```python
from build123d import *

# Parameters (mm, degrees)
SKETCH1_R               = 2
BOSS_EXTRUDE1_DEPTH     = 6
SKETCH1_3_W             = 26
SKETCH1_3_H             = 13
BOSS_EXTRUDE2_DEPTH     = 32
FILLET1_R               = 2.5
SKETCH2_R               = 9
CUT_EXTRUDE1_DEPTH      = 42.221960167
CUT_EXTRUDE2_REACH      = 48.971
CUT_EXTRUDE2_END_RADIUS = 9
SKETCH3_R               = 2
FILLET2_R               = 1


with BuildPart() as part:
    # Sketch1 → Boss-Extrude1 (new body)
    with BuildSketch(Plane(origin=(0, 0, 0), x_dir=(1, 0, 0), z_dir=(0, 1, 0))):
        with BuildLine():
            Line((-13, 0), (-22.5, 0))
            Line((-22.5, 0), (-22.5, -21))
            ThreePointArc((-22.5, -21), (-21.035533906, -24.535533906), (-17.5, -26))
            Line((-17.5, -26), (17.5, -26))
            ThreePointArc((17.5, -26), (21.035533906, -24.535533906), (22.5, -21))
            Line((22.5, -21), (22.5, 0))
            Line((22.5, 0), (13, 0))
            Line((13, 0), (13, -13))
            Line((13, -13), (-13, -13))
            Line((-13, -13), (-13, 0))
        make_face()
        with Locations(Location((0, -19.5, 0), (0, 0, 270))):
            Circle(SKETCH1_R, mode=Mode.SUBTRACT)
        with Locations(Location((-18, -6.5, 0), (0, 0, 270))):
            Circle(SKETCH1_R, mode=Mode.SUBTRACT)
        with Locations(Location((18, -6.5, 0), (0, 0, 270))):
            Circle(SKETCH1_R, mode=Mode.SUBTRACT)
    extrude(amount=BOSS_EXTRUDE1_DEPTH)

    # Sketch1<3> → Boss-Extrude2 (add)
    with BuildSketch(Plane(origin=(0, 0, 0), x_dir=(1, 0, 0), z_dir=(0, 1, 0))):
        with Locations((0, -6.5)):
            Rectangle(SKETCH1_3_W, SKETCH1_3_H)
    extrude(amount=BOSS_EXTRUDE2_DEPTH)

    # Fillet1
    fillet1_edges = [part.edges().sort_by_distance(p)[0] for p in [
        (-13, 32, 6.5),
        (13, 32, 6.5),
    ]]
    fillet(fillet1_edges, radius=FILLET1_R)

    # Sketch2 → Cut-Extrude1 (cut, through all)
    with BuildSketch(Plane.XY.offset(13)):
        with Locations((0, 19)):
            Circle(SKETCH2_R)
    extrude(amount=-CUT_EXTRUDE1_DEPTH, mode=Mode.SUBTRACT)

    # Cut-Extrude2: up to this cylinder (the profile starts outside it)
    cut_extrude2_end = Plane(origin=(0, 19, 6.5), z_dir=(0, 0, 1)) * Cylinder(CUT_EXTRUDE2_END_RADIUS, 116.942, mode=Mode.PRIVATE)
    # Sketch3 → Cut-Extrude2 (cut, up to the surface)
    with BuildSketch(Plane(origin=(0, 32, 0), x_dir=(1, 0, 0), z_dir=(0, 1, 0)), mode=Mode.PRIVATE) as cut_extrude2_sk1:
        with Locations(Location((0, -6.5, 0), (0, 0, 270))):
            Circle(SKETCH3_R)
    cut_extrude2_tool1 = extrude(cut_extrude2_sk1.sketch, amount=-CUT_EXTRUDE2_REACH, mode=Mode.PRIVATE) - cut_extrude2_end
    add(cut_extrude2_tool1.solids().sort_by_distance((0, 32, 6.5))[0], mode=Mode.SUBTRACT)

    # Fillet2
    fillet2_edges = [part.edges().sort_by_distance(p)[0] for p in [
        (13, 6, 6.5),
        (0, 6, 13),
        (-13, 6, 6.5),
    ]]
    fillet(fillet2_edges, radius=FILLET2_R)


solid = part.part
```
Geometry check sheet. Reference: the model listing, model coordinates, mm. A direction names the side the tool comes from. Round coordinates to 2 decimals unless told otherwise and drop trailing zeros. Loops run counter-clockwise (first coordinate to the right, second up) from the corner with the lowest first, then second, coordinate; pieces in that order, holes last. Notation, with made-up numbers: (32.25, 47) - (68.25, 47) arc R18 cw to (68.25, 66) - close; hole circle Ø3 at (33.5, 21.5). An arc over 180 degrees is marked (long way). Use a Markdown table: item, result.
Q1. Cross-section at C-C on x = 0. Record the cut outline in (y, z), plus the area to 3 significant figures.
Solutions:
| item | result |
|---|---|
| outline | (0, 0) - (10, 0) - (10, 13) - (7, 13) arc R1 cw to (6, 14) - (6, 17.5) - (0, 17.5) - close; (0, 21.5) - (6, 21.5) - (6, 26) - (0, 26) - close; (28, 0) - (32, 0) - (32, 4.5) - (28, 4.5) - close; (28, 8.5) - (32, 8.5) - (32, 13) - (28, 13) - close |
| area | 220 mm2 |
Q2. Cross-section at D-D on z = 19.5. Record the cut outline in (x, y).
Solutions:
| item | result |
|---|---|
| outline | (-22.5, 0) - (-2, 0) - (-2, 6) - (-22.5, 6) - close; (2, 0) - (22.5, 0) - (22.5, 6) - (2, 6) - close |
Q3. Cross-section at A-A on y = 19. Record the cut outline in (x, z).
Solutions:
| item | result |
|---|---|
| outline | (-13, 0) - (-9, 0) - (-9, 13) - (-13, 13) - close; (9, 0) - (13, 0) - (13, 13) - (9, 13) - close |
Q4. Go/stop test with flat-tipped pins: P1, Ø1.5, axis at y = 25.5, z = 8, coming from the +X side; P2, Ø10.5, axis at y = 14, z = 6.5, coming from the -X side; P3, Ø3.5, axis at x = -18, z = 6.5, coming from the -Y side; P4, Ø5, axis at x = -16, z = 13.5, coming from the +Y side. Record where each tip stops, or that it passes through.
Solutions:
| item | result |
|---|---|
| P1 | stops at x = 13 |
| P2 | stops at x = -13 |
| P3 | passes through |
| P4 | stops at y = 6.13 |
Q5. Cross-section at B-B on z = 6.5. Record the cut outline in (x, y), plus the area to 3 significant figures.
Solutions:
| item | result |
|---|---|
| outline | (-22.5, 0) - (-20, 0) - (-20, 6) - (-22.5, 6) - close; (-16, 0) - (16, 0) - (16, 6) - (14, 6) arc R1 cw to (13, 7) - (13, 29.5) arc R2.5 ccw to (10.5, 32) - (2, 32) - (2, 27.77) arc R9 cw (long way) to (-2, 27.77) - (-2, 32) - (-10.5, 32) arc R2.5 ccw to (-13, 29.5) - (-13, 7) arc R1 cw to (-14, 6) - (-16, 6) - close; (20, 0) - (22.5, 0) - (22.5, 6) - (20, 6) - close |
| area | 625 mm2 |
Q6. Access from +Z, -Z, +X, -X, +Y, -Y to the whole of each face (thin tool, end or side, straight path). Record for faces 5 (the cylindrical face through (-12.287, 31.248, 6.409)), 6 (the flat face through (-3, 28, 13)), 7 (the flat face through (0, 6, 16)), 8 (the cylindrical face through (-1.2, 29.9, 4.9)).
Solutions:
| item | result |
|---|---|
| face 5 | +Z, -Z, -X, +Y |
| face 6 | +Z, +X, -X, +Y |
| face 7 | +Z, +Y |
| face 8 | +Y |
Q7. Material ranges on line 1 (X direction, y = 3.6, z = 6.5); line 2 (Y direction, x = 0, z = 10); line 3 (X direction, y = 8, z = 12.5), recorded low to high.
Solutions:
| item | result |
|---|---|
| line 1 | x = -22.5 to -20, -16 to 16, 20 to 22.5 |
| line 2 | y = 0 to 10, 28 to 32 |
| line 3 | x = -13 to 13 |
Q8. Draft check along X on faces 1 (the cylindrical face through (19.983, 2.958, 6.24)), 2 (the flat face through (0, 0, 13)), 3 (the cylindrical face through (13.301, 6.285, 7.098)), 4 (the cylindrical face through (-21.07, 2.96, 24.5)). Enter one of: released by +X, released by -X, zero draft, split by the parting line, or undercut.
Solutions:
| item | result |
|---|---|
| face 1 | undercut |
| face 2 | zero draft |
| face 3 | released by +X |
| face 4 | released by -X |
